Solid Edge part; units mm, degrees
sketch "Sketch1" plane through (0, 0, 0) normal (0, 0, 1) x (1, 0, 0)
  line L0 (-1.55, 15.85) -> (-3.7, 15.85)
  line L1 (-3.7, 15.85) -> (-3.7, -15.85)
  line L2 (-3.7, -15.85) -> (-1.55, -15.85)
  arc A0 (-1.55, -15.85) -> (4, -10.3) centre (-1.55, -10.3) ccw
  line L3 (4, -10.3) -> (4, 10.3)
  arc A1 (-1.55, 15.85) -> (4, 10.3) centre (-1.55, 10.3) cw
  line L4 (-1.5, 20) -> (-7.7, 20)
  line L5 (-7.7, 20) -> (-7.7, -20)
  line L6 (-7.7, -20) -> (-1.5, -20)
  arc A2 (7.5, -11) -> (-1.5, -20) centre (-1.5, -11) cw
  line L7 (7.5, -11) -> (7.5, 11)
  arc A3 (-1.5, 20) -> (7.5, 11) centre (-1.5, 11) cw
extrude "Protrusion1" add sketch "Sketch1" along normal blind 4
sketch "Sketch2" plane through (0, 0, 0) normal (0, 0, 1) x (1, 0, 0)
  arc A0 (-37.7, -20) -> (-49.7, -8) centre (-37.7, -8) cw
  line L0 (-49.7, 8) -> (-49.7, -8)
  arc A1 (-37.7, 20) -> (-49.7, 8) centre (-37.7, 8) ccw
  line L1 (-7.7, 20) -> (-37.7, 20)
  line L2 (-7.7, 20) -> (-7.7, -20)
  line L3 (-37.7, -20) -> (-7.7, -20)
extrude "ProtrusiónExtruida_7" add sketch "Sketch2" along normal blind 4
sketch "Sketch3" plane through (0, 0, 0) normal (0, 0, 1) x (1, 0, 0)
  line L0 (-3.7, -15.85) -> (-1.55, -15.85)
  arc A0 (-1.55, -15.85) -> (4, -10.3) centre (-1.55, -10.3) ccw
  line L1 (4, -10.3) -> (4, 10.3)
  arc A1 (-1.55, 15.85) -> (4, 10.3) centre (-1.55, 10.3) cw
  line L2 (-1.55, 15.85) -> (-3.7, 15.85)
  line L3 (-3.7, 15.85) -> (-3.7, -15.85)
extrude "ProtrusiónExtruida_8" add sketch "Sketch3" along normal blind 12
CAD build for the part. Positions are in the model's coordinates, mm. A direction names the side the tool comes from. Coordinates: 2 decimals unless noted, no trailing zeros. Loops run counter-clockwise (first coordinate to the right, second up) from the corner with the lowest first, then second, coordinate; pieces in that order, holes last. Notation, with made-up numbers: (32, 76.5) -> (85, 76.5) arc R32 ccw to (85, 106.5) -> close; hole circle Ø6 at (-8.5, 39). An arc over 180 degrees is marked (long way). One line per item, written item: value.
1. Slice it at D-D on z = 8.75. Write the cut outline in (x, y).
Answers:
outline: (-3.7, -15.85) -> (-1.55, -15.85) arc R5.55 ccw to (4, -10.3) -> (4, 10.3) arc R5.55 ccw to (-1.55, 15.85) -> (-3.7, 15.85) -> close
2. Which spindle directions (+Z, -Z, +X, -X, +Y, -Y) get a long thin tool onto all of the face, cutting with end or side? Do faces 1 (the face through (4, 0, 8)), 2 (the face through (2.3, 14.3, 7.9)), 3 (the face through (2.4, -14.2, 7.9)). Say none if no direction does.
Answers:
face 1: +Z, +X, +Y, -Y
face 2: +Z, +X, +Y
face 3: +Z, +X, -Y
3. Flat gauge pins, fed straight in: P1, Ø1.7, axis at x = -3, z = 8.5, coming from the +Y side; P2, Ø5, axis at y = 2, z = 7.5, coming from the -X side; P3, Ø2.5, axis at y = -1.5, z = 9, coming from the +X side; P4, Ø4, axis at x = -10, z = 7.5, coming from the -Y side. Where does each tip first touch, or does it go through?
Answers:
P1: stops at y = 15.85
P2: stops at x = -3.7
P3: stops at x = 4
P4: passes through
4. Slice it at C-C on x = -9. Write the cut outline in (y, z), and give its area (3 significant figures).
Answers:
outline: (-20, 0) -> (20, 0) -> (20, 4) -> (-20, 4) -> close
area: 160 mm^2
5. Slice it at A-A on y = 3. Write the cut outline in (x, z), and give its area (3 significant figures).
Answers:
outline: (-49.7, 0) -> (7.5, 0) -> (7.5, 4) -> (4, 4) -> (4, 12) -> (-3.7, 12) -> (-3.7, 4) -> (-49.7, 4) -> close
area: 290 mm^2
6. Drill centre lines: line 1 (X direction, y = 9, z = 5.25); line 2 (Z direction, x = -39.5, y = -8); line 3 (X direction, y = -10, z = 0.5). Where is each one in solid material? Low to high. Write a range as [from, to].
Answers:
line 1: x = [-3.7, 4]
line 2: z = [0, 4]
line 3: x = [-49.53, 7.5]
7. Slice it at B-B on z = 1. Write the cut outline in (x, y), and give its area (3 significant figures).
Answers:
outline: (-49.7, -8) arc R12 ccw to (-37.7, -20) -> (-1.5, -20) arc R9 ccw to (7.5, -11) -> (7.5, 11) arc R9 ccw to (-1.5, 20) -> (-37.7, 20) arc R12 ccw to (-49.7, 8) -> close
area: 2,190 mm^2
